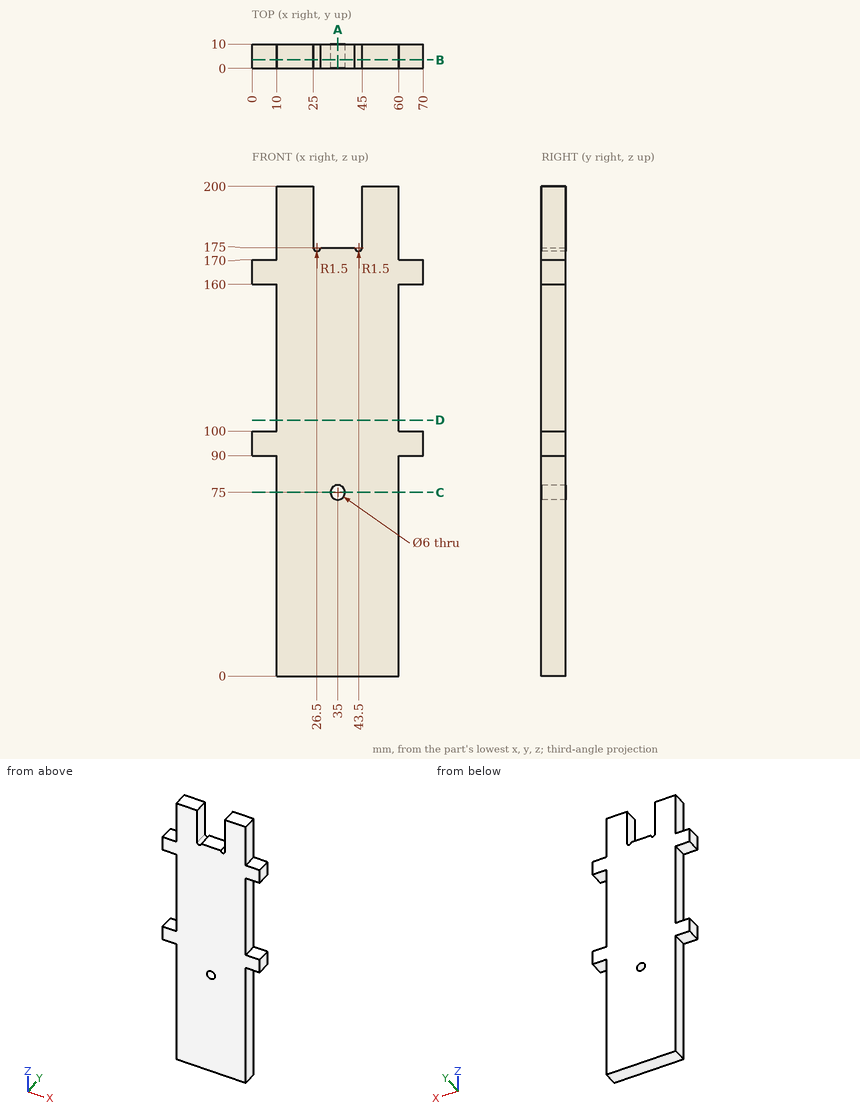
Could you check a few things on this drawing? It's one solid part, dimensions in mm from its lowest x, y, z. Give positions to 0.01 mm unless a question says otherwise; leave off trailing zeros. Loops run counter-clockwise (first coordinate to the right, second up) from the corner with the lowest first, then second, coordinate; pieces in that order, holes last. Notation, with made-up numbers: M -0.5,52 L 58.5,52 A13 cw 58.5,68 Z; hole C 29,53 d1. An arc over 180 degrees is marked long. Return JSON: item names as keys, results as strings.
Item 1: Imagine slicing it at B-B on y = 3.5. List the corners of the cut face in (x, z) for me.
A:
{"outline": "M 0,90 L 10,90 L 10,0 L 60,0 L 60,90 L 70,90 L 70,100 L 60,100 L 60,160 L 70,160 L 70,170 L 60,170 L 60,200 L 45,200 L 45,175 A1.5 cw 42,175 L 28,175 A1.5 cw 25,175 L 25,200 L 10,200 L 10,170 L 0,170 L 0,160 L 10,160 L 10,100 L 0,100 Z; hole C 35,75 d6"}
Item 2: Imagine slicing it at A-A on x = 35. List the corners of the cut face in (y, z) for me, then the cut area to 3 significant figures.
A:
{"outline": "M 0,0 L 10,0 L 10,72 L 0,72 Z; M 0,78 L 10,78 L 10,175 L 0,175 Z", "area": "1,690 mm^2"}
Item 3: Imagine slicing it at C-C on z = 75. List the corners of the cut face in (x, y) for me, then the cut area to 3 significant figures.
A:
{"outline": "M 10,0 L 32,0 L 32,10 L 10,10 Z; M 38,0 L 60,0 L 60,10 L 38,10 Z", "area": "440 mm^2"}
Item 4: I'm going to push flat-ended pins straight in: pin 1 Ø5 at (x, y) = (3.5, 7) entering from +Z; pin 2 Ø3 at (x, y) = (6.5, 3.5) entering from -Z; pin 3 Ø2 at (y, z) = (4, 56.5) entering from -X; pin 4 Ø5 at (y, z) = (1.5, 161) entering from -X. Where does each tip first touch, or does it pass through?
A:
{"pin 1": "stops at z = 170", "pin 2": "stops at z = 90", "pin 3": "stops at x = 10", "pin 4": "stops at x = 0"}
Item 5: Please list where these lines run through material, in increasing order: line 1 (Z direction, x = 35, y = 6); line 2 (Z direction, x = 66.5, y = 0.75); line 3 (X direction, y = 8.75, z = 106.5).
A:
{"line 1": "z = 0 to 72, 78 to 175", "line 2": "z = 90 to 100, 160 to 170", "line 3": "x = 10 to 60"}
Item 6: Imagine slicing it at D-D on z = 104.5. List the corners of the cut face in (x, y) for me, then the cut area to 3 significant figures.
A:
{"outline": "M 10,0 L 60,0 L 60,10 L 10,10 Z", "area": "500 mm^2"}
